Autodesk Inventor part; units mm, degrees
ref_plane "YZ Plane" through (0, 0, 0) normal (1, 0, 0) x (0, 1, 0)
ref_plane "XZ Plane" through (0, 0, 0) normal (0, 1, 0) x (-1, 0, 0)
ref_plane "XY Plane" through (0, 0, 0) normal (0, 0, 1) x (1, 0, 0)
sketch "Sketch1" plane through (0, 0, 0) normal (1, 0, 0) x (0, 1, 0)
  circle A0 centre (143.9084, 246.9114) radius 25.4 construction
  circle A1 centre (165.3998, 156.5759) radius 25.4 construction
  circle A2 centre (143.9084, 246.9114) radius 14.2875
  circle A3 centre (165.3998, 156.5759) radius 14.2875
  arc A4 (180.8102, 358.5299) -> (124.0141, 358.5299) centre (152.4121, 333.1299) ccw
  line L0 (127.0121, 361.528) -> (111.7556, 346.2715)
  line L1 (151.8132, 8.702) -> (48.4022, 8.702)
  line L2 (117.9037, 202.8627) -> (109.9063, 341.4154)
  arc A5 (111.7556, 346.2715) -> (109.9063, 341.4154) centre (116.2457, 341.7813) ccw
  arc A6 (116.7471, 198.8279) -> (117.9037, 202.8627) centre (111.5643, 202.4968) ccw
  arc A7 (151.8132, 8.702) -> (158.0642, 13.9355) centre (151.8132, 15.052) ccw
  circle A8 centre (44.0062, 25.4424) radius 14.2875
  line L3 (48.4022, 8.702) -> (25.3949, 8.702)
  line L4 (180.8102, 358.5299) -> (219.6983, 334.9834)
  line L5 (222.7593, 329.5515) -> (222.7593, 222.4129)
  line L6 (222.4715, 220.5229) -> (158.0642, 13.9355)
  arc A9 (222.7593, 329.5515) -> (219.6983, 334.9834) centre (216.4093, 329.5515) ccw
  arc A10 (222.4715, 220.5229) -> (222.7593, 222.4129) centre (216.4093, 222.4129) ccw
  circle A11 centre (196.3745, 222.9354) radius 14.2875
  circle A12 centre (196.3745, 197.5354) radius 2.5781
  circle A13 centre (196.3745, 248.3354) radius 2.5781
  line L7 (25.3949, 111.9383) -> (116.7471, 198.8279)
  line L8 (25.3949, 8.702) -> (25.3949, 111.9383)
  circle A14 centre (145.8462, 22.3213) radius 6.35
  point P0 (177.8121, 361.528)
  dimension "d2" = 28.575
  dimension "d3" = 28.575
  dimension "d18" = 6.35
  dimension "d19" = 28.575
  dimension "d21" = 5.1562
  dimension "d36" = 12.7
extrude "Extrusion1" add sketch "Sketch1" along normal blind 9.525 contours L4 A9 L5 A10 L6 A7 L1 L3 L8 L7 A6 L2 A5 L0 A4
properties part number "Intake-v1"
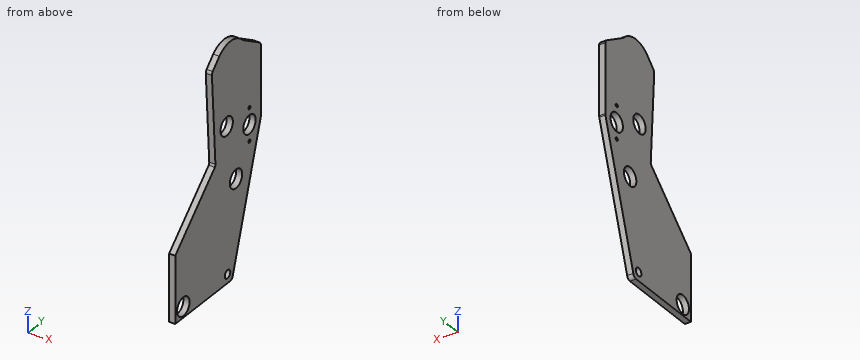
Could you check a few things on this model? Use its own coordinates, in mm. Give positions to 0.01 mm unless a question says otherwise; leave off trailing zeros. Write each loop counter-clockwise with the first axis right and the second up, starting at its lowest first coordinate (ties: lowest second). Pieces come first, ordered by that corner, then holes. Notation, with made-up numbers: (80.25, 63.25) -> (131.25, 63.25) arc R23 cw to (131.25, 90.25) -> close; hole circle Ø8 at (70, -23). An arc over 180 degrees is marked (long way). Write each question's results on one line, items separated by ' | '. Start each with the question number.
Q1. Suppose I cut it at D-D, the plane z = 81. List the corners of the cut face in (x, y) for me (3 decimals), and give its area (3 significant figures).
Q2. I need wall thicknesses on probe 1 along Z at (x, y) = (6.5, 156); probe 2 along Y at (x, z) = (8.5, 223); probe 3 along Z at (x, y) = (1.5, 141.5). Which ranges of each line are inside material? Lowest first, please.
Q3. Suppose I cut it at A-A, the plane z = 153. List the corners of the cut face in (x, y) for me (1 decimal).
Q4. I'm going to push flat-ended pins straight in: pin 1 Ø6 at (y, z) = (196.37, 197.54) entering from +X (3 decimals); pin 2 Ø5 at (x, z) = (8.5, 333) entering from -Y; pin 3 Ø2 at (x, z) = (6.5, 84) entering from +Y; pin 4 Ø4 at (x, y) = (6, 200.5) entering from +Z. Where does each tip first touch, or does it pass through?
Q5. Suppose I cut it at B-B, the plane x = 8. State how many separate pieces and enclosed holes the cut face has, and give its area (3 significant figures).
Q6. Suppose I cut it at C-C, the plane y = 190. List the corners of the cut face in (x, z) for me (3 decimals), and give its area (3 significant figures).
Outcome:
1) outline: (0, 25.395) -> (9.525, 25.395) -> (9.525, 178.973) -> (0, 178.973) -> close | area: 1,460 mm2
2) probe 1: 10.28 to 145.82, 167.34 to 239.3, 254.52 to 371.06 | probe 2: 116.74 to 182.09, 210.66 to 222.76 | probe 3: 8.7 to 17.69, 26.95 to 232.83, 260.99 to 369.63
3) outline: (0, 68.6) -> (9.5, 68.6) -> (9.5, 151.6) -> (0, 151.6) -> close; (0, 179.2) -> (9.5, 179.2) -> (9.5, 201.4) -> (0, 201.4) -> close
4) pin 1: x = 9.525 | pin 2: y = 110.25 | pin 3: y = 180.22 | pin 4: z = 347.82
5) separate pieces: 1 | enclosed holes: 7 | area: 41,100 mm2
6) outline: (0, 116.37) -> (9.525, 116.37) -> (9.525, 210.149) -> (0, 210.149) -> close; (0, 235.722) -> (9.525, 235.722) -> (9.525, 352.966) -> (0, 352.966) -> close | area: 2,010 mm2
